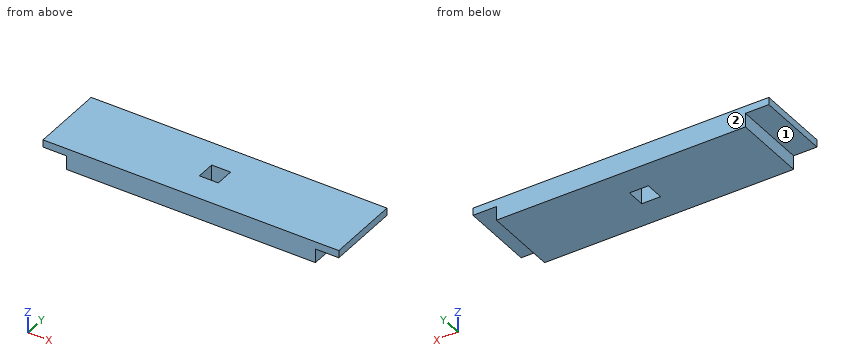
from build123d import *

# Parameters (mm, degrees)
SKETCH1_W           = 254
SKETCH1_H           = 63.5
BOSS_EXTRUDE1_DEPTH = 18.288
SKETCH2_W           = 16.2052
SKETCH2_H           = 16.2052
CUT_EXTRUDE1_DEPTH  = 263.455140822
SKETCH3_W           = 20.066
SKETCH3_H           = 63.5
CUT_EXTRUDE2_DEPTH  = 11.938


with BuildPart() as part:
    # Sketch1 → Boss-Extrude1 (new body)
    with BuildSketch(Plane.XY):
        with Locations((127, 31.75)):
            Rectangle(SKETCH1_W, SKETCH1_H)
    extrude(amount=BOSS_EXTRUDE1_DEPTH)

    # Sketch2 → Cut-Extrude1 (cut, through all)
    with BuildSketch(Plane.XY.offset(18.288)):
        with Locations((127, 31.75)):
            Rectangle(SKETCH2_W, SKETCH2_H)
    extrude(amount=-CUT_EXTRUDE1_DEPTH, mode=Mode.SUBTRACT)

    # Sketch3 → Cut-Extrude2 (cut)
    with BuildSketch(Plane(origin=(0, 0, 0), x_dir=(-1, 0, 0), z_dir=(0, 0, -1))):
        with Locations((-243.967, 31.75)):
            Rectangle(SKETCH3_W, SKETCH3_H)
        with Locations((-10.033, 31.75)):
            Rectangle(SKETCH3_W, SKETCH3_H)
    extrude(amount=-CUT_EXTRUDE2_DEPTH, mode=Mode.SUBTRACT)


solid = part.part
Here's how the part is built. I have some questions about the finished solid (model axes, mm). Face numbers are marked on the shaded views. A direction names the side the tool comes from. Give positions to 0.01 mm unless a question says otherwise; leave off trailing zeros. Order: outer loops, then holes, each group sorted by start corner. A loop starts at its lowest first (then second) coordinate and runs counter-clockwise, first axis right, second up. Notation, with made-up numbers: (20, 69) -> (43, 69) arc R23 cw to (43, 89) -> close; hole circle Ø9 at (-21, 10). An arc over 180 degrees is marked (long way). One line per item, written item: value. Start each with the question number.
1. Imagine slicing it at A-A, the plane z = 3.25. List the corners of the cut face in (x, y) for me.
2. I need wall thicknesses on probe 1 along X at (y, z) = (30.5, 12); probe 2 along Y at (x, z) = (130.5, 4.75); probe 3 along X at (y, z) = (14.5, 2). Which ranges of each line are inside material? Lowest first, please. Write a range as from..to.
3. Imagine slicing it at B-B, the plane y = 27. List the corners of the cut face in (x, z) for me.
4. For the marked faces 1 and 2, which set-ups out of +Z, -Z, +X, -X, +Y, -Y let a thin tool reach every point of the face, with its end or its side?
5. Will these pins go through, and if not, where does the flat tip stop? pin 1 Ø1.5 at (y, z) = (19, 10.5) entering from +X; pin 2 Ø1 at (y, z) = (20.5, 6.5) entering from -X; pin 3 Ø10 at (x, y) = (11.5, 35) entering from -Z.
6. Imagine slicing it at D-D, the plane z = 15.75. List the corners of the cut face in (x, y) for me, plus the area to 3 significant figures.
7. Imagine slicing it at C-C, the plane y = 11.5. List the corners of the cut face in (x, z) for me.
Values follow:
1. outline: (20.07, 0) -> (233.93, 0) -> (233.93, 63.5) -> (20.07, 63.5) -> close; hole (118.9, 23.65) -> (135.1, 23.65) -> (135.1, 39.85) -> (118.9, 39.85) -> close
2. probe 1: x = 0..118.9, 135.1..254
2. probe 2: y = 0..23.65, 39.85..63.5
2. probe 3: x = 20.07..233.93
3. outline: (0, 11.94) -> (20.07, 11.94) -> (20.07, 0) -> (118.9, 0) -> (118.9, 18.29) -> (0, 18.29) -> close; (135.1, 0) -> (233.93, 0) -> (233.93, 11.94) -> (254, 11.94) -> (254, 18.29) -> (135.1, 18.29) -> close
4. face 1: -Z, -X, +Y, -Y
4. face 2: +Z, -Z, +X, -X, +Y
5. pin 1: stops at x = 233.93
5. pin 2: stops at x = 20.07
5. pin 3: stops at z = 11.94
6. outline: (0, 0) -> (254, 0) -> (254, 63.5) -> (0, 63.5) -> close; hole (118.9, 23.65) -> (135.1, 23.65) -> (135.1, 39.85) -> (118.9, 39.85) -> close
6. area: 15,900 mm2
7. outline: (0, 11.94) -> (20.07, 11.94) -> (20.07, 0) -> (233.93, 0) -> (233.93, 11.94) -> (254, 11.94) -> (254, 18.29) -> (0, 18.29) -> close
